Can you work these out from the model? Positions are in its coordinate system, mm. A direction names the side the tool comes from. Round coordinates to 2 decimals unless told otherwise and drop trailing zeros. Loops run counter-clockwise (first coordinate to the right, second up) from the corner with the lowest first, then second, coordinate; pieces in that order, holes last.
from build123d import *
from build123d.topology import SkipClean

# Parameters (mm, degrees)
BOSS_EXTRUDE1_DEPTH = 5
BOSS_EXTRUDE2_START = -10
BOSS_EXTRUDE2_DEPTH = 10
SKETCH4_W           = 100
SKETCH4_H           = 79
CUT_EXTRUDE1_DEPTH  = 30
BOSS_EXTRUDE3_DEPTH = 37
SKETCH8_W           = 5
SKETCH8_H           = 79
BOSS_EXTRUDE6_DEPTH = 100
FILLET3_R           = 6.1
FILLET4_R           = 6.1
BOSS_EXTRUDE7_DEPTH = 5
SKETCH10_W          = 5
SKETCH10_H          = 32
BOSS_EXTRUDE8_DEPTH = 5
SKETCH11_W          = 32
SKETCH11_H          = 5
BOSS_EXTRUDE9_DEPTH = 5
FILLET6_R           = 1


with BuildPart() as part:
    # Sketch1 → Boss-Extrude1 (new body)
    with BuildSketch(Plane.XY):
        with BuildLine():
            Line((-57.206320908, 108.379254457), (110.593679092, 108.379254457))
            ThreePointArc((110.593679092, 108.379254457), (114.907030458, 106.592605822), (116.693679092, 102.279254457))
            Line((116.693679092, 102.279254457), (116.693679092, -65.520745543))
            ThreePointArc((116.693679092, -65.520745543), (114.907030458, -69.834096908), (110.593679092, -71.620745543))
            Line((110.593679092, -71.620745543), (-57.206320908, -71.620745543))
            ThreePointArc((-57.206320908, -71.620745543), (-61.519672273, -69.834096908), (-63.306320908, -65.520745543))
            Line((-63.306320908, -65.520745543), (-63.306320908, 102.279254457))
            ThreePointArc((-63.306320908, 102.279254457), (-61.519672273, 106.592605822), (-57.206320908, 108.379254457))
        make_face()
    extrude(amount=BOSS_EXTRUDE1_DEPTH)

    # Sketch3 → Boss-Extrude2 (add)
    with SkipClean():  # the faces are left unmerged after this step: merging them gives an invalid solid
        with BuildSketch(Plane.XY.offset(5).offset(BOSS_EXTRUDE2_START)):
            with BuildLine():
                ThreePointArc((-57.206320908, 108.379254457), (-61.519672273, 106.592605822), (-63.306320908, 102.279254457))
                Line((-63.306320908, 102.279254457), (-63.306320908, -65.520745543))
                ThreePointArc((-63.306320908, -65.520745543), (-61.519672273, -69.834096908), (-57.206320908, -71.620745543))
                Line((-57.206320908, -71.620745543), (110.593679092, -71.620745543))
                ThreePointArc((110.593679092, -71.620745543), (114.907030458, -69.834096908), (116.693679092, -65.520745543))
                Line((116.693679092, -65.520745543), (116.693679092, 102.279254457))
                ThreePointArc((116.693679092, 102.279254457), (114.907030458, 106.592605822), (110.593679092, 108.379254457))
                Line((110.593679092, 108.379254457), (-57.206320908, 108.379254457))
            make_face()
            with BuildLine():
                Line((105.593338585, -66.620625471), (-52.206661415, -66.620625471))
                ThreePointArc((-52.206661415, -66.620625471), (-56.520012781, -64.833976836), (-58.306661415, -60.520625471))
                Line((-58.306661415, -60.520625471), (-58.306661415, 97.279374529))
                ThreePointArc((-58.306661415, 97.279374529), (-56.520012781, 101.592725894), (-52.206661415, 103.379374529))
                Line((-52.206661415, 103.379374529), (105.593338585, 103.379374529))
                ThreePointArc((105.593338585, 103.379374529), (109.90668995, 101.592725894), (111.693338585, 97.279374529))
                Line((111.693338585, 97.279374529), (111.693338585, -60.520625471))
                ThreePointArc((111.693338585, -60.520625471), (109.90668995, -64.833976836), (105.593338585, -66.620625471))
            make_face(mode=Mode.SUBTRACT)
        extrude(amount=BOSS_EXTRUDE2_DEPTH)
    add(part.part.scale(1), mode=Mode.REPLACE)  # the faces are merged on a copy

    # Sketch4 → Cut-Extrude1 (cut, symmetric)
    with BuildSketch(Plane.XY.offset(5)):
        with Locations((-13.306320908, 68.879254457)):
            Rectangle(SKETCH4_W, SKETCH4_H)
    extrude(amount=CUT_EXTRUDE1_DEPTH, both=True, mode=Mode.SUBTRACT)

    # Sketch5 → Boss-Extrude3 (add)
    with BuildSketch(Plane.XY.offset(5)):
        with BuildLine():
            Line((36.693679092, 108.379254457), (41.693679092, 108.379254457))
            Line((41.693679092, 108.379254457), (41.693679092, 30.479254457))
            ThreePointArc((41.693679092, 30.479254457), (39.907030458, 26.165903092), (35.593679092, 24.379254457))
            Line((35.593679092, 24.379254457), (-63.306320908, 24.379254457))
            Line((-63.306320908, 24.379254457), (-63.306320908, 29.379254457))
            Line((-63.306320908, 29.379254457), (30.593679092, 29.379254457))
            ThreePointArc((30.593679092, 29.379254457), (34.907030458, 31.165903092), (36.693679092, 35.479254457))
            Line((36.693679092, 35.479254457), (36.693679092, 108.379254457))
        make_face()
    extrude(amount=-BOSS_EXTRUDE3_DEPTH)

    # Sketch8 → Boss-Extrude6 (add)
    with BuildSketch(Plane.ZY.offset(-36.693679092)):
        with Locations((-29.5, 68.879254457)):
            Rectangle(SKETCH8_W, SKETCH8_H)
    extrude(amount=BOSS_EXTRUDE6_DEPTH)

    # Fillet3
    fillet3_edges = [part.edges().sort_by_distance(p)[0] for p in [
        (-63.306320908, 108.379254457, -29.5),
    ]]
    fillet(fillet3_edges, radius=FILLET3_R)

    # Fillet4
    fillet4_edges = [part.edges().sort_by_distance(p)[0] for p in [
        (34.907030458, 31.165903092, -27),
        (36.693679092, 71.929254457, -27),
        (-16.356320908, 29.379254457, -27),
    ]]
    fillet(fillet4_edges, radius=FILLET4_R)

    # Sketch9 → Boss-Extrude7 (add)
    with BuildSketch(Plane(origin=(0, 0, -32), x_dir=(-1, 0, 0), z_dir=(0, 0, -1))):
        with BuildLine():
            Line((-41.693679092, 103.379254457), (52.206342763, 103.379254457))
            ThreePointArc((52.206342763, 103.379254457), (56.519684701, 101.592615249), (58.306342763, 97.279281121))
            Line((58.306342763, 97.279281121), (58.306661415, 24.379254457))
            Line((58.306661415, 24.379254457), (63.306661415, 24.379254457))
            Line((63.306661415, 24.379254457), (63.306320908, 102.279254457))
            ThreePointArc((63.306320908, 102.279254457), (61.519672273, 106.592605822), (57.206320908, 108.379254457))
            Line((57.206320908, 108.379254457), (-41.693679092, 108.379254457))
            Line((-41.693679092, 108.379254457), (-41.693679092, 103.379254457))
        make_face()
    extrude(amount=BOSS_EXTRUDE7_DEPTH)

    # Sketch10 → Boss-Extrude8 (add)
    with BuildSketch(Plane.XZ.offset(-24.379254457)):
        with Locations((-60.806661415, -21)):
            Rectangle(SKETCH10_W, SKETCH10_H)
    extrude(amount=BOSS_EXTRUDE8_DEPTH)

    # Sketch11 → Boss-Extrude9 (add)
    with BuildSketch(Plane(origin=(41.693679092, 0, 0), x_dir=(0, 0, -1), z_dir=(1, 0, 0))):
        with Locations((21, 105.879254457)):
            Rectangle(SKETCH11_W, SKETCH11_H)
    extrude(amount=BOSS_EXTRUDE9_DEPTH)

    # Fillet6
    fillet6_edges = [part.edges().sort_by_distance(p)[0] for p in [
        (73.643508838, 103.379374529, 0),
        (-11.356491162, 24.379254457, 0),
        (39.907030458, 26.165903092, 0),
        (41.693679092, 66.929314493, 0),
        (41.693679092, 66.929254457, -32),
        (39.907030458, 26.165903092, -32),
        (-11.356491162, 24.379254457, -32),
        (-60.806661415, 19.379254457, -37),
        (-60.806491162, 19.379254457, -5),
        (-58.306661415, -18.070685507, 0),
        (46.693679092, 105.879254457, -37),
        (46.693679092, 105.879314493, -5),
        (109.90668995, 101.592725894, 0),
        (111.693338585, 18.379374529, 0),
        (109.90668995, -64.833976836, 0),
        (26.693338585, -66.620625471, 0),
        (-56.520012781, -64.833976836, 0),
    ]]
    fillet(fillet6_edges, radius=FILLET6_R)


solid = part.part
(1) If we section it at D-D, the plane x = 58: List the corners of the cut face in (y, z) for me, then the cut area to 3 significant figures.
Worked answers:
outline: (-71.62, -5) - (-66.62, -5) - (-66.62, -1) arc R1 cw to (-65.62, 0) - (102.38, 0) arc R1 cw to (103.38, -1) - (103.38, -5) - (108.38, -5) - (108.38, 5) - (-71.62, 5) - close
area: 950 mm2
(2) If we mould it in two halves opening along X, with no side actions, what happens to faces 1 (the flat face through (-63.306, 13, -4)), 2 (the flat face through (39, 108.379, -17)), 3 (the flat face through (111.693, 19, -3))? For each: released by +X, released by -X, zero draft, split by the parting line, or undercut.
Worked answers:
face 1: released by -X
face 2: zero draft
face 3: undercut
(3) For faces 4 (the flat face through (46, -68, -5)), 5 (the flat face through (28, -66.621, -3)), 6 (the flat face through (-61, 19.379, -20)), 7 (the cylindrical face through (-15.699, 31.214, -25.261)), 8 (the cylindrical face through (115, 106.5, -0.1)), which set-ups out of +Z, -Z, +X, -X, +Y, -Y let a thin tool reach every point of the face, with its end or its side?
Worked answers:
face 4: -Z, +X, -Y
face 5: -Z
face 6: -Z, +X, -X, -Y
face 7: +Z, -X, +Y
face 8: +Z, -Z, +X, +Y
(4) If I drill on line 1 (Y direction, x = 24, z = -2.5); line 2 (X direction, y = 92, z = -7.5); line 3 (Z direction, x = -49.5, y = 49.5), over which ranges is the centre line in solid material (lowest first)?
Worked answers:
line 1: y = -71.62 to -66.62, 24.38 to 29.38
line 2: x = 36.69 to 41.69
line 3: z = -32 to -27
(5) Will these pins go through, and if not, where does the flat tip stop? P1, Ø5.5, axis at x = -60.5, z = -20, coming from the -Y side; P2, Ø1, axis at x = -9.5, z = -5.5, coming from the +Y side; P3, Ø3, axis at y = 18, z = -9.5, coming from the +X side; P4, Ø18, axis at y = -26.5, z = -15.5, coming from the +X side.
Worked answers:
P1: stops at y = 19.38
P2: stops at y = 29.38
P3: stops at x = -58.31
P4: passes through
(6) If we section it at A-A, the plane y = -57.5: List the corners of the cut face in (x, z) for me, then the cut area to 3 significant figures.
Worked answers:
outline: (-63.31, -5) - (-58.31, -5) - (-58.31, -1) arc R1 cw to (-57.31, 0) - (110.69, 0) arc R1 cw to (111.69, -1) - (111.69, -5) - (116.69, -5) - (116.69, 5) - (-63.31, 5) - close
area: 950 mm2
(7) If we section it at B-B, the plane x = -24.5: List the corners of the cut face in (y, z) for me.
Worked answers:
outline: (-71.62, -5) - (-66.62, -5) - (-66.62, -1) arc R1 cw to (-65.62, 0) - (23.38, 0) arc R1 cw to (24.38, -1) - (24.38, -31) arc R1 ccw to (25.38, -32) - (103.38, -32) - (103.38, -37) - (108.38, -37) - (108.38, -27) - (35.48, -27) arc R6.1 cw to (29.38, -20.9) - (29.38, 5) - (-71.62, 5) - close
